```python
from build123d import *

# Parameters (mm, degrees)
PAD_DEPTH       = 5
SKETCH001_W     = 150
SKETCH001_H     = 5
PAD001_DEPTH    = 50
SKETCH002_W     = 150
SKETCH002_H     = 4
PAD002_DEPTH    = 60
SKETCH003_W     = 150
SKETCH003_H     = 4
PAD003_DEPTH    = 20
SKETCH004_W     = 68
SKETCH004_H     = 19
PAD004_DEPTH    = 35
SKETCH005_W     = 60
SKETCH005_H     = 13
POCKET_DEPTH    = 35
SKETCH006_R     = 2.1
POCKET001_DEPTH = 5
CHAMFER_SIZE    = 2


with BuildPart() as part:
    # Sketch → Pad (new body)
    with BuildSketch(Plane.XY):
        Polygon((0, 0), (0, 95), (70, 165), (80, 165), (150, 95), (150, 0), align=None)
    extrude(amount=PAD_DEPTH)

    # Sketch001 (on Face8 of Pad) → Pad001 (join)
    with BuildSketch(Plane.XY.offset(5)):
        with Locations((75, 2.5)):
            Rectangle(SKETCH001_W, SKETCH001_H)
    extrude(amount=PAD001_DEPTH)

    # Sketch002 (on Face11 of Pad001) → Pad002 (join)
    with BuildSketch(Plane(origin=(0, 5, 0), x_dir=(-1, 0, 0), z_dir=(0, 1, 0))):
        with Locations((-75, 18)):
            Rectangle(SKETCH002_W, SKETCH002_H)
    extrude(amount=PAD002_DEPTH)

    # Sketch003 (on Face10 of Pad002) → Pad003 (join)
    with BuildSketch(Plane(origin=(0, 5, 0), x_dir=(-1, 0, 0), z_dir=(0, 1, 0))):
        with Locations((-75, 53)):
            Rectangle(SKETCH003_W, SKETCH003_H)
    extrude(amount=PAD003_DEPTH)

    # Sketch004 (on Face10 of Pad003) → Pad004 (join)
    with BuildSketch(Plane(origin=(0, 5, 0), x_dir=(-1, 0, 0), z_dir=(0, 1, 0))):
        with Locations((-34, 41.5)):
            Rectangle(SKETCH004_W, SKETCH004_H)
    extrude(amount=PAD004_DEPTH)

    # Sketch005 (on Face23 of Pad004) → Pocket (cut)
    with BuildSketch(Plane(origin=(0, 40, 0), x_dir=(-1, 0, 0), z_dir=(0, 1, 0))):
        with Locations((-34, 41.5)):
            Rectangle(SKETCH005_W, SKETCH005_H)
    extrude(amount=-POCKET_DEPTH, mode=Mode.SUBTRACT)

    # Sketch006 (on Face5 of Pocket) → Pocket001 (cut)
    with BuildSketch(Plane.XY.offset(5)):
        with Locations((75, 158)):
            Circle(SKETCH006_R)
    extrude(amount=-POCKET001_DEPTH, mode=Mode.SUBTRACT)

    # Chamfer
    chamfer_edges = [part.edges().sort_by_distance(p)[0] for p in [
        (72.9, 158, 5),
    ]]
    chamfer(chamfer_edges, length=CHAMFER_SIZE)


solid = part.part
```
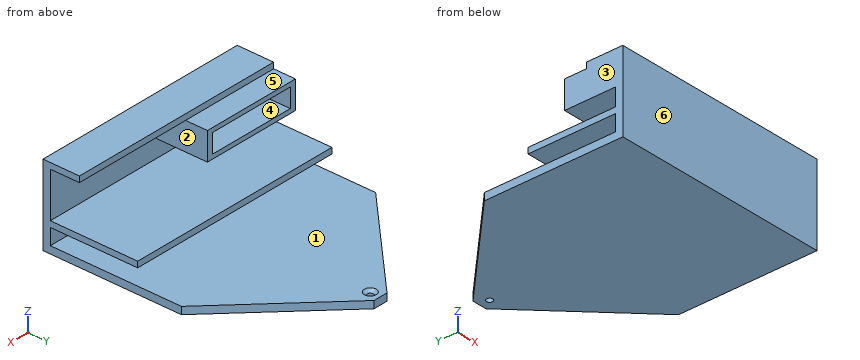
Verification items for the finished model (mm, model axes). Face numbers are marked on the shaded views. A direction names the side the tool comes from. Coordinates: 2 decimals unless noted, no trailing zeros. Write each loop counter-clockwise with the first axis right and the second up, starting at its lowest first coordinate (ties: lowest second). Pieces come first, ordered by that corner, then holes. Notation, with made-up numbers: M 11.25,64 L 31.25,64 A19 ccw 31.25,69 Z; hole C 61,48 d1. An arc over 180 degrees is marked long. Answer as a JSON object with one key per item and string values. Group by question number.
(1) Gauge pin test, flat ends, axial feed: pin 1 (4.5 mm diameter, centred on x = 35.5, y = 30, fed in from +Z); pin 2 (6.5 mm diameter, centred on y = 27, z = 39, fed in from -X); pin 3 (4 mm diameter, centred on y = 22.5, z = 43, fed in from +X); pin 4 (1 mm diameter, centred on x = 53, z = 20, fed in from +Y). Record the tip position at first contact, or that the pin passes through.
(2) Cross-section at A-A, the plane y = 14.5. Record the cut outline in (x, z), and give its area (3 significant figures).
(3) Material ranges on line 1 (Z direction, x = 47.5, y = 13); line 2 (Y direction, x = 75, z = 1); line 3 (Z direction, x = 112, y = 20.5), recorded low to high.
(4) Cross-section at C-C, the plane y = 61. Record the cut outline in (x, z).
(5) Cross-section at B-B, the plane x = 75. Record the cut outline in (y, z).
(6) Release check for a two-part mould opening along Z. For the marked faces 4, 5 and 6 record: +Z half, -Z half, draft (parallel to the pull), parting line (faces both ways), or undercut.
(7) Tool access check on the marked faces 1, 2 and 3. Record the directions out of +Z, -Z, +X, -X, +Y, -Y that give a thin tool (end or side, any length) a straight path to the whole face; none if there is none.
(8) Cross-section at D-D, the plane x = 35. Record the cut outline in (y, z), and give its area (3 significant figures).
Reply:
{
 "1": {"pin 1": "z = 51", "pin 2": "x = 0", "pin 3": "x = 68", "pin 4": "y = 65"},
 "2": {"outline": "M 0,0 L 150,0 L 150,5 L 0,5 Z; M 0,16 L 150,16 L 150,20 L 0,20 Z; M 0,32 L 68,32 L 68,51 L 150,51 L 150,55 L 0,55 Z; hole M 4,35 L 64,35 L 64,48 L 4,48 Z", "area": "2,460 mm²"},
 "3": {"line 1": "0 to 5, 16 to 20, 32 to 35, 48 to 55", "line 2": "0 to 155.9, 160.1 to 165", "line 3": "0 to 5, 16 to 20, 51 to 55"},
 "4": {"outline": "M 0,0 L 150,0 L 150,5 L 0,5 Z; M 0,16 L 150,16 L 150,20 L 0,20 Z"},
 "5": {"outline": "M 0,0 L 155.9,0 L 155.9,3 L 153.9,5 L 5,5 L 5,16 L 65,16 L 65,20 L 5,20 L 5,51 L 25,51 L 25,55 L 0,55 Z; M 160.1,0 L 165,0 L 165,5 L 162.1,5 L 160.1,3 Z"},
 "6": {"face 4": "undercut", "face 5": "+Z half", "face 6": "draft"},
 "7": {"face 1": "+X, -X, +Y", "face 2": "+X, +Y", "face 3": "+Z, -Z, -X, +Y, -Y"},
 "8": {"outline": "M 0,0 L 130,0 L 130,5 L 5,5 L 5,16 L 65,16 L 65,20 L 5,20 L 5,32 L 40,32 L 40,35 L 5,35 L 5,48 L 40,48 L 40,51 L 25,51 L 25,55 L 0,55 Z", "area": "1,430 mm²"}
}
